```python
from build123d import *

# Parameters (mm, degrees)
BOSS_EXTRUDE1_DEPTH = 20
CHAMFER1_SIZE       = 2.5
SKETCH2_R           = 7.5
CUT_EXTRUDE1_DEPTH  = 85.852813742
CUT_EXTRUDE2_DEPTH  = 60
CUT_EXTRUDE3_DEPTH  = 85.852813742
CHAMFER2_SIZE       = 1


with BuildPart() as part:
    # Sketch1 → Boss-Extrude1 (new body)
    with BuildSketch(Plane.XY):
        Polygon((0, 0), (0, 20), (20, 20), (20, 10), (80, 5), (80, 0), align=None)
    extrude(amount=BOSS_EXTRUDE1_DEPTH)

    # Chamfer1
    chamfer1_edges = [part.edges().sort_by_distance(p)[0] for p in [
        (50, 7.5, 20),
        (50, 7.5, 0),
    ]]
    chamfer(chamfer1_edges, length=CHAMFER1_SIZE)

    # Sketch2 → Cut-Extrude1 (cut, through all)
    with BuildSketch(Plane(origin=(0, 0, 0), x_dir=(-1, 0, 0), z_dir=(0, -1, 0))):
        with Locations(Location((-10, -10, 0), (0, 0, 90))):
            Circle(SKETCH2_R)
    extrude(amount=-CUT_EXTRUDE1_DEPTH, mode=Mode.SUBTRACT)

    # Sketch3 → Cut-Extrude2 (cut)
    with BuildSketch(Plane(origin=(80, 0, 0), x_dir=(0, 0, -1), z_dir=(1, 0, 0))):
        Polygon((-15, 2.199704526), (-16.27, 0), (-13.73, 0), align=None)
        Polygon((-6.27, 0), (-5, 2.199704526), (-3.73, 0), align=None)
    extrude(amount=-CUT_EXTRUDE2_DEPTH, mode=Mode.SUBTRACT)

    # Sketch4 → Cut-Extrude3 (cut, through all)
    with BuildSketch(Plane.XY):
        Polygon((75, 2.199704526), (73.73, 0), (76.27, 0), align=None)
        Polygon((65, 2.199704526), (63.73, 0), (66.27, 0), align=None)
        Polygon((50, 2.199704526), (48.73, 0), (51.27, 0), align=None)
        Polygon((35, 2.199704526), (33.73, 0), (36.27, 0), align=None)
    extrude(amount=CUT_EXTRUDE3_DEPTH, mode=Mode.SUBTRACT)

    # Chamfer2
    chamfer2_edges = [part.edges().sort_by_distance(p)[0] for p in [
        (10, 20, 17.5),
        (10, 0, 17.5),
    ]]
    chamfer(chamfer2_edges, length=CHAMFER2_SIZE)


solid = part.part
```
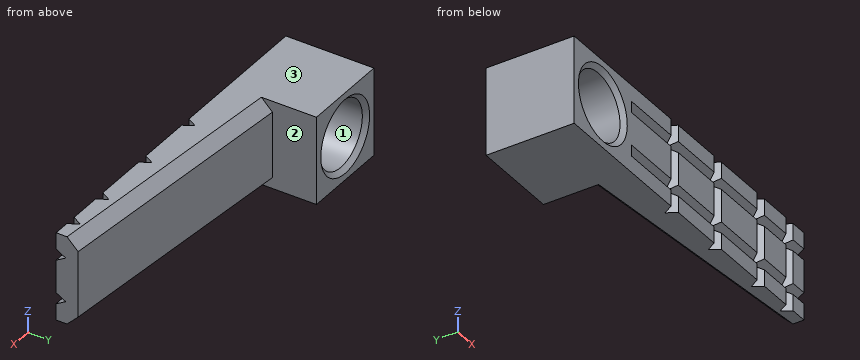
For this review, take the finished solid that the model builds, in its own axes (mm). Face numbers are marked on the shaded views. Round coordinates to 2 decimals unless told otherwise and drop trailing zeros. Order: outer loops, then holes, each group sorted by start corner. A loop starts at its lowest first (then second) coordinate and runs counter-clockwise, first axis right, second up.
Q1. We need section A-A, the plane x = 10. Give the boundary of the cut face in (y, z).
Findings below:
outline: (0, 0) - (20, 0) - (20, 1.5) - (19, 2.5) - (1, 2.5) - (0, 1.5) - close; (0, 18.5) - (1, 17.5) - (19, 17.5) - (20, 18.5) - (20, 20) - (0, 20) - close
Q2. Insertion check: P1, Ø6, axis at x = 46, y = 12, coming from the +Z side; P2, Ø0.7, axis at y = 1, z = 15, coming from the +X side; P3, Ø5, axis at x = 58.5, z = 10.5, coming from the +Y side; P4, Ø8, axis at x = 47.5, z = 12.5, coming from the +Y side. Each pin has a flat end and moves straight along its axis. Give the tip position at first contact, or say it passes through.
Findings below:
P1: passes through
P2: stops at x = 20
P3: stops at y = 7
P4: stops at y = 8.04
Q3. We need section B-B, the plane z = 10. Give the boundary of the cut face in (x, y), plus the area to 3 significant figures.
Findings below:
outline: (0, 0) - (1.5, 0) - (2.5, 1) - (2.5, 19) - (1.5, 20) - (0, 20) - close; (17.5, 1) - (18.5, 0) - (33.73, 0) - (35, 2.2) - (36.27, 0) - (48.73, 0) - (50, 2.2) - (51.27, 0) - (63.73, 0) - (65, 2.2) - (66.27, 0) - (73.73, 0) - (75, 2.2) - (76.27, 0) - (80, 0) - (80, 5) - (20, 10) - (20, 20) - (18.5, 20) - (17.5, 19) - close
area: 537 mm2
Q4. We need section D-D, the plane x = 46.5. Give the boundary of the cut face in (y, z).
Findings below:
outline: (0, 0) - (5.28, 0) - (7.79, 2.5) - (7.79, 17.5) - (5.28, 20) - (0, 20) - (0, 16.27) - (2.2, 15) - (0, 13.73) - (0, 6.27) - (2.2, 5) - (0, 3.73) - close
Q5. Mouldability with a two-part tool opening along Z and no side actions: class the marked faces 1, 2 and 3 as pulls with the +Z half, pulls with the -Z half, needs draft (parallel to the pull), parting line crosses it, or undercut.
Findings below:
face 1: undercut
face 2: needs draft
face 3: pulls with the +Z half
Q6. Wall thickness on line 1 (X direction, y = 16, z = 3.5); line 2 (X direction, y = 12.5, z = 10); line 3 (X direction, y = 1.25, z = 19.25): over which ranges is each line inside the solid? List them lowest first.
Findings below:
line 1: x = 0 to 6.26, 13.74 to 20
line 2: x = 0 to 2.5, 17.5 to 20
line 3: x = 0 to 34.45, 35.55 to 49.45, 50.55 to 64.45, 65.55 to 74.45, 75.55 to 80
Q7. We need section C-C, the plane x = 57. Give the boundary of the cut face in (y, z).
Findings below:
outline: (0, 0) - (4.41, 0) - (6.92, 2.5) - (6.92, 17.5) - (4.41, 20) - (0, 20) - (0, 16.27) - (2.2, 15) - (0, 13.73) - (0, 6.27) - (2.2, 5) - (0, 3.73) - close
